Read the model definition and answer for the solid it produces. Units are mm, in the model's axes. Face numbers are marked on the shaded views. A direction names the side the tool comes from. Coordinates: 2 decimals unless noted, no trailing zeros. Write each loop counter-clockwise with the first axis right and the second up, starting at its lowest first coordinate (ties: lowest second). Pieces come first, ordered by that corner, then holes. Notation, with made-up numbers: (68, 25) -> (127, 25) arc R30 cw to (127, 54) -> close; hole circle Ø1 at (62.25, 88.25). An arc over 180 degrees is marked (long way). Use CSV: the item, a comma, the result in double quotes.
Autodesk Inventor part; units mm, degrees
ref_plane "YZ Plane" through (0, 0, 0) normal (1, 0, 0) x (0, 1, 0)
ref_plane "XZ Plane" through (0, 0, 0) normal (0, 1, 0) x (-1, 0, 0)
ref_plane "XY Plane" through (0, 0, 0) normal (0, 0, 1) x (1, 0, 0)
sketch "Esquisse2" plane through (0, 0, 0) normal (0, 1, 0) x (-1, 0, 0)
  circle A0 centre (0, 0) radius 7.2
  dimension "d0" = 14.4
extrude "Extrusion1" add sketch "Esquisse2" along normal blind 15
sketch "Esquisse4" plane through (0, 15, 0) normal (0, 1, 0) x (1, 0, 0)
  circle A0 centre (0, 0) radius 7.2
  circle A1 centre (0, 0) radius 7.2
  arc A2 (-2, -6.9166) -> (0, -7.2) centre (0, 0) ccw
  arc A3 (-1.4444, -4.9954) -> (0, -5.2) centre (0, 0) ccw
  line L0 (-2, -6.9166) -> (-1.4444, -4.9954)
  line L1 (0, -7.2) -> (0, -5.2)
  line L2 (0, 0) -> (-4.1531, -9.129)
  arc A4 (-5.4277, -4.7308) -> (-3.9, -6.0523) centre (0, 0) ccw
  arc A5 (-3.92, -3.4167) -> (-2.8167, -4.3711) centre (0, 0) ccw
  line L3 (-3.9, -6.0523) -> (-2.8167, -4.3711)
  line L4 (-5.4277, -4.7308) -> (-3.92, -3.4167)
  line L5 (0, -6) -> (0, 5.5969) construction
  line L6 (0, 0) -> (-5.5895, -3.594)
  arc A6 (-6.5507, 2.988) -> (-7.1229, 1.0507) centre (0, 0) ccw
  arc A7 (-4.7311, 2.158) -> (-5.1443, 0.7589) centre (0, 0) ccw
  line L7 (-7.1229, 1.0507) -> (-5.1443, 0.7589)
  line L8 (-6.5507, 2.988) -> (-4.7311, 2.158)
  arc A8 (-7.125, -1.0366) -> (-6.5566, -2.975) centre (0, 0) ccw
  arc A9 (-5.1458, -0.7487) -> (-4.7353, -2.1486) centre (0, 0) ccw
  line L9 (-7.125, -1.0366) -> (-5.1458, -0.7487)
  line L10 (-6.5566, -2.975) -> (-4.7353, -2.1486)
  line L11 (-2, -6.9166) -> (-3.9, -6.0523) construction
  line L12 (-5.4277, -4.7308) -> (-6.5566, -2.975) construction
  line L13 (-2, -6.9166) -> (0, -7.2) construction
  line L14 (0, 0) -> (-5.7368, 3.7048)
  arc A10 (-3.888, 6.06) -> (-5.4183, 4.7415) centre (0, 0) ccw
  line L15 (-5.4183, 4.7415) -> (-3.9132, 3.4244)
  line L16 (-3.888, 6.06) -> (-2.808, 4.3767)
  arc A11 (-2.808, 4.3767) -> (-3.9132, 3.4244) centre (0, 0) ccw
  line L17 (-1.9863, 6.9206) -> (-1.4345, 4.9982)
  arc A12 (0.0143, 7.2) -> (-1.9863, 6.9206) centre (0, 0) ccw
  arc A13 (0.0103, 5.2) -> (-1.4345, 4.9982) centre (0, 0) ccw
  line L18 (0.0143, 7.2) -> (0.0103, 5.2)
  line L19 (-6.5507, 2.988) -> (-5.4183, 4.7415) construction
  line L20 (0, 0) -> (1.7786, 11.975)
  arc A14 (1.9726, -6.9245) -> (3.8184, -6.1041) centre (0, 0) ccw
  arc A15 (1.4246, -5.001) -> (2.7578, -4.4085) centre (0, 0) ccw
  line L21 (1.9726, -6.9245) -> (1.4246, -5.001)
  line L22 (3.8184, -6.1041) -> (2.7578, -4.4085)
  arc A16 (7.1208, -1.0648) -> (7.1364, 0.9551) centre (0, 0) ccw
  line L23 (7.1364, 0.9551) -> (5.154, 0.6898)
  line L24 (7.1208, -1.0648) -> (5.1428, -0.7691)
  arc A17 (5.1428, -0.7691) -> (5.154, 0.6898) centre (0, 0) ccw
  line L25 (6.5161, -3.0627) -> (4.7061, -2.212)
  arc A18 (5.4089, -4.7522) -> (6.5161, -3.0627) centre (0, 0) ccw
  arc A19 (3.9064, -3.4322) -> (4.7061, -2.212) centre (0, 0) ccw
  line L26 (5.4089, -4.7522) -> (3.9064, -3.4322)
  line L27 (3.8184, -6.1041) -> (5.4089, -4.7522) construction
  line L28 (2.079, 6.8933) -> (1.5015, 4.9785)
  arc A20 (2.8253, 4.3655) -> (1.5015, 4.9785) centre (0, 0) ccw
  line L29 (3.912, 6.0445) -> (2.8253, 4.3655)
  arc A21 (3.912, 6.0445) -> (2.079, 6.8933) centre (0, 0) ccw
  arc A22 (4.7396, 2.1392) -> (3.9588, 3.3716) centre (0, 0) ccw
  line L30 (5.4815, 4.6684) -> (3.9588, 3.3716)
  line L31 (6.5625, 2.962) -> (4.7396, 2.1392)
  arc A23 (6.5625, 2.962) -> (5.4815, 4.6684) centre (0, 0) ccw
  line L32 (7.1364, 0.9551) -> (6.5625, 2.962) construction
  line L33 (0.0143, 7.2) -> (2.079, 6.8933) construction
  point P0 (3.8184, -6.1041)
  point P1 (6.5161, -3.0627)
  point P2 (7.1208, -1.0648)
  point P3 (7.1364, 0.9551)
  point P4 (5.4815, 4.6684)
  point P5 (2.079, 6.8933)
  point P6 (-6.5507, 2.988)
  point P7 (-7.1229, 1.0507)
  point P8 (-6.5566, -2.975)
  point P9 (-2, -6.9166)
  point P10 (0, -7.2)
  point P11 (-5.4277, -4.7308)
  point P12 (-3.9, -6.0523)
  dimension "d13" = 2
  dimension "d14" = 2
  dimension "d16" = 1.9
extrude "Extrusion2" cut sketch "Esquisse4" against normal through all contours A0 L24 A17 L23 | L31 A22 L30 A0 | A0 L26 A19 L25 | L29 A20 L28 A0 | A0 L21 A15 L22 | A0 L0 A3 L1 | L18 A13 L17 A0 | L16 A11 L15 A0 | A0 L4 A5 L3 | L8 A7 L7 A0 | A0 L9 A9 L10
sketch "Esquisse5" plane through (0, 15, 0) normal (0, 1, 0) x (1, 0, 0)
  point P0 (0, 0)
sketch "Esquisse6" plane through (0, 15, 0) normal (0, 1, 0) x (1, 0, 0)
  circle A0 centre (0, 0) radius 8
  dimension "d19" = 16
extrude "Extrusion3" add sketch "Esquisse6" along normal blind 1.5
sketch "Esquisse7" plane through (0, 0, 0) normal (0, -1, 0) x (1, 0, 0)
  circle A0 centre (0, 0) radius 8
extrude "Extrusion4" add sketch "Esquisse7" along normal blind 1.5
sketch "Esquisse8" plane through (0, 16.5, 0) normal (0, 1, 0) x (1, 0, 0)
  circle A0 centre (0, 0) radius 4
  dimension "d24" = 8
extrude "Extrusion5" cut sketch "Esquisse8" against normal through all
properties part number "Pièce_moteur_courroie_test_1"
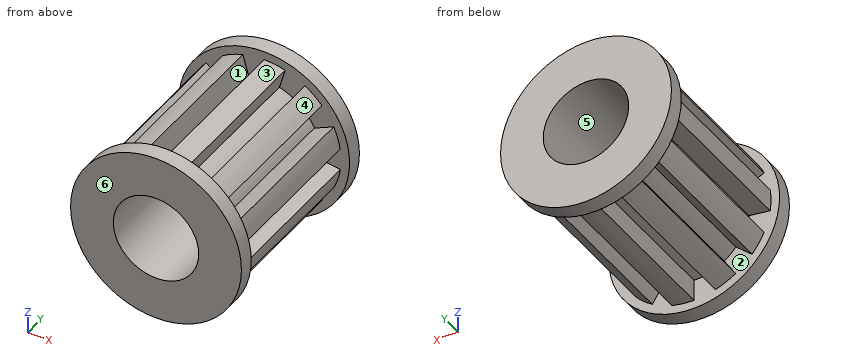
1. A cutting plane is placed at A-A (z = 0). Give the vertices of the cut face in (x, y), and give its area (3 significant figures).
Solutions:
outline,"(-8, -1.5) -> (-4, -1.5) -> (-4, 16.5) -> (-8, 16.5) -> (-8, 15) -> (-7.2, 15) -> (-7.2, 0) -> (-8, 0) -> close; (4, -1.5) -> (8, -1.5) -> (8, 0) -> (5.2, 0) -> (5.2, 15) -> (8, 15) -> (8, 16.5) -> (4, 16.5) -> close"
area,"90.0 mm^2"
2. Each of these flat-tipped pins is pushed along its axis until it touches: pin 1 Ø1 at (x, y) = (-3.5, 11.5) entering from +Z; pin 2 Ø6 at (y, z) = (8, 5) entering from +X; pin 3 Ø1.6 at (y, z) = (4, 6) entering from -X; pin 4 Ø7 at (x, z) = (0, 0) entering from +Y. Where does it stop, or does it pass through?
Solutions:
pin 1,"stops at z = 6.55"
pin 2,"stops at x = 6.92"
pin 3,"stops at x = -3.9"
pin 4,"passes through"
3. A tool of negligible diameter and unlimited length cuts with its end or side. For the marked faces 1, 2 and 3, from which of +Z, -Z, +X, -X, +Y, -Y can it reach the whole face along a straight path? Write none if from no direction.
Solutions:
face 1,"+Z"
face 2,"none"
face 3,"+Z, +X"
4. For a pull along Y with two mould halves and no side action, classify the marked faces 4, 5 and 6 as pulls with the +Y half, pulls with the -Y half, needs draft (parallel to the pull), parting line crosses it, or undercut.
Solutions:
face 4,"undercut"
face 5,"needs draft"
face 6,"pulls with the -Y half"
5. A cutting plane is placed at B-B (x = 6.25). Give the vertices of the cut face in (y, z).
Solutions:
outline,"(-1.5, -4.99) -> (0, -4.99) -> (0, -2.82) -> (15, -2.82) -> (15, -4.99) -> (16.5, -4.99) -> (16.5, 4.99) -> (15, 4.99) -> (15, 2.94) -> (0, 2.94) -> (0, 4.99) -> (-1.5, 4.99) -> close; hole (0, -0.84) -> (15, -0.84) -> (15, 0.93) -> (0, 0.93) -> close"
6. Find the intervals of material crossed by line 1 along Y through (x, z) = (-7.5, -2.5); line 2 along X through (y, z) = (13.5, 5.75); line 3 along Z through (x, y) = (-5.25, 7.75), in increasing order.
Solutions:
line 1,"y = -1.5 to 0, 15 to 16.5"
line 2,"x = -3.71 to -1.66, 0 to 1.64, 3.6 to 4.33"
line 3,"z = -4.59 to -2.39, -0.77 to 0.76, 2.38 to 4.58"
7. A cutting plane is placed at D-D (z = 5.5). Give the vertices of the cut face in (x, y).
Solutions:
outline,"(-5.81, -1.5) -> (5.81, -1.5) -> (5.81, 0) -> (4.65, 0) -> (4.65, 15) -> (5.81, 15) -> (5.81, 16.5) -> (-5.81, 16.5) -> (-5.81, 15) -> (-3.54, 15) -> (-3.54, 0) -> (-5.81, 0) -> close; hole (-1.59, 0) -> (0, 0) -> (0, 15) -> (-1.59, 15) -> close; hole (1.57, 0) -> (3.44, 0) -> (3.44, 15) -> (1.57, 15) -> close"
8. A cutting plane is placed at C-C (x = 4.25). Give the vertices of the cut face in (y, z), and give its area (3 significant figures).
Solutions:
outline,"(-1.5, -6.78) -> (0, -6.78) -> (0, -5.81) -> (15, -5.81) -> (15, -6.78) -> (16.5, -6.78) -> (16.5, 6.78) -> (15, 6.78) -> (15, 5.81) -> (0, 5.81) -> (0, 6.78) -> (-1.5, 6.78) -> close; hole (0, -3.62) -> (15, -3.62) -> (15, -3) -> (0, -3) -> close; hole (0, 3) -> (15, 3) -> (15, 3.73) -> (0, 3.73) -> close"
area,"195 mm^2"
